from build123d import *

# Parameters (mm, degrees)
SKETCH1_W                    = 235
SKETCH1_H                    = 1200
BASE_FLANGE1_DEPTH           = 1
EDGE_FLANGE2_STRIP_W         = 5.4732
EDGE_FLANGE2_STRIP_H         = 1
EDGE_FLANGE2_STRIP_CUT_DEPTH = 1200
EDGE_FLANGE2_DEPTH           = 1200
EDGE_FLANGE3_DEPTH           = 1200
EDGE_FLANGE4_STRIP_W         = 5.4732
EDGE_FLANGE4_STRIP_H         = 1
EDGE_FLANGE4_STRIP_CUT_DEPTH = 1200
EDGE_FLANGE4_DEPTH           = 1200
EDGE_FLANGE5_DEPTH           = 1200


# Sheet-metal steps are written as plain solids
with BuildPart() as part:
    # Sketch1 → Base-Flange1 (new body)
    with BuildSketch(Plane.XY):
        with Locations((-1020.895638629, 1263.161993769)):
            Rectangle(SKETCH1_W, SKETCH1_H)
    extrude(amount=-BASE_FLANGE1_DEPTH)

    # Edge-Flange2 strip (across the edge) → Edge-Flange2 strip cut (cut)
    with BuildSketch(Plane(origin=(-1138.395638629, 1863.161993769, 0), x_dir=(1, 0, 0), z_dir=(0, -1, 0))):
        with Locations((-1, -0.5)):
            Rectangle(EDGE_FLANGE2_STRIP_W, EDGE_FLANGE2_STRIP_H)
    extrude(amount=EDGE_FLANGE2_STRIP_CUT_DEPTH, mode=Mode.SUBTRACT)

    # Edge-Flange2 section (across the edge) → Edge-Flange2 (add)
    with BuildSketch(Plane(origin=(-1138.395638629, 1863.161993769, 0), x_dir=(1, 0, 0), z_dir=(0, -1, 0))):
        with BuildLine():
            Line((0, 0.7366), (0, 51))
            Line((0, 51), (1, 51))
            Line((1, 51), (1, 0.7366))
            ThreePointArc((1, 0.7366), (1.215745145, 0.215745145), (1.7366, 0))
            Line((1.7366, 0), (1.7366, -1))
            ThreePointArc((1.7366, -1), (0.508638364, -0.491361636), (0, 0.7366))
        make_face()
    extrude(amount=EDGE_FLANGE2_DEPTH)

    # Edge-Flange3 section (across the edge) → Edge-Flange3 (add)
    with BuildSketch(Plane(origin=(-1137.395638629, 1863.161993769, 51.7366), x_dir=(0, 0, -1), z_dir=(0, -1, 0))):
        with BuildLine():
            Line((-1, 0.7366), (-1, 14))
            Line((-1, 14), (0, 14))
            Line((0, 14), (0, 0.7366))
            ThreePointArc((0, 0.7366), (0.215745145, 0.215745145), (0.7366, 0))
            Line((0.7366, 0), (0.7366, -1))
            ThreePointArc((0.7366, -1), (-0.491361636, -0.491361636), (-1, 0.7366))
        make_face()
    extrude(amount=EDGE_FLANGE3_DEPTH)

    # Edge-Flange4 strip (across the edge) → Edge-Flange4 strip cut (cut)
    with BuildSketch(Plane(origin=(-903.395638629, 663.161993769, 0), x_dir=(-1, 0, 0), z_dir=(0, 1, 0))):
        with Locations((-1, -0.5)):
            Rectangle(EDGE_FLANGE4_STRIP_W, EDGE_FLANGE4_STRIP_H)
    extrude(amount=EDGE_FLANGE4_STRIP_CUT_DEPTH, mode=Mode.SUBTRACT)

    # Edge-Flange4 section (across the edge) → Edge-Flange4 (add)
    with BuildSketch(Plane(origin=(-903.395638629, 663.161993769, 0), x_dir=(-1, 0, 0), z_dir=(0, 1, 0))):
        with BuildLine():
            Line((0, 0.7366), (0, 67))
            Line((0, 67), (1, 67))
            Line((1, 67), (1, 0.7366))
            ThreePointArc((1, 0.7366), (1.215745145, 0.215745145), (1.7366, 0))
            Line((1.7366, 0), (1.7366, -1))
            ThreePointArc((1.7366, -1), (0.508638364, -0.491361636), (0, 0.7366))
        make_face()
    extrude(amount=EDGE_FLANGE4_DEPTH)

    # Edge-Flange5 section (across the edge) → Edge-Flange5 (add)
    with BuildSketch(Plane(origin=(-904.395638629, 663.161993769, 67.7366), x_dir=(0, 0, -1), z_dir=(0, 1, 0))):
        with BuildLine():
            Line((-1, 0.7366), (-1, 49))
            Line((-1, 49), (0, 49))
            Line((0, 49), (0, 0.7366))
            ThreePointArc((0, 0.7366), (0.215745145, 0.215745145), (0.7366, 0))
            Line((0.7366, 0), (0.7366, -1))
            ThreePointArc((0.7366, -1), (-0.491361636, -0.491361636), (-1, 0.7366))
        make_face()
    extrude(amount=EDGE_FLANGE5_DEPTH)


solid = part.part
Input: part model. Units: mm. Frame: model coordinates. A direction names the side the tool comes from. Give positions to 0.01 mm unless a question says otherwise; leave off trailing zeros. Write each loop counter-clockwise with the first axis right and the second up, starting at its lowest first coordinate (ties: lowest second). Pieces come first, ordered by that corner, then holes.
Q1. Set-up query: faces 1 (the face through (-930, 1255, 67.737)), 2 (the face through (-903.396, 1255, 33)), 3 (the face through (-1023, 1272, 0)). Return all of +Z, -Z, +X, -X, +Y, -Y with unobstructed straight access to the full face (end or side cutting, diameter ignored); none if empty.
Q2. Section A-A, the plane z = 38.5. Output: boundary loops of the cut face in (x, y), plus the area to 3 significant figures.
Q3. Section D-D, the plane x = -1006. Output: boundary loops of the cut face in (y, z).
Q4. First-contact query: P1, Ø4, axis at x = -1130, y = 1096, coming from the +Z side; P2, Ø10, axis at x = -1057.5, y = 1654.5, coming from the +Z side; P3, Ø1, axis at y = 1635, z = 55.5, coming from the -X side. Flat tips, straight axial feed; report the tip coordinate or a pass-through.
Q5. Pull-direction query (Z, two-part tool) for faces 4 (the face through (-1138.396, 1272, 26)), 5 (the face through (-929, 1255, 68.737)), 6 (the face through (-1137.396, 1272, 26)); classes: pulls with the +Z half, pulls with the -Z half, needs draft (parallel to the pull), parting line crosses it, or undercut.
Q6. Section B-B, the plane x = -943. Output: boundary loops of the cut face in (y, z).
Q7. Section C-C, the plane y = 1551.5. Output: boundary loops of the cut face in (x, z).
Q8. Material intervals for probe 1 along Z at (x, y) = (-932.5, 1653.5); probe 2 along X at (y, z) = (1348.5, 38.5); probe 3 along Z at (x, y) = (-1070, 1383.5), sorted ascending.
Filled in:
1. face 1: -X, +Y, -Y
1. face 2: +Z, -Z, +X, +Y, -Y
1. face 3: +Y, -Y
2. outline: (-1138.4, 663.16) - (-1137.4, 663.16) - (-1137.4, 1863.16) - (-1138.4, 1863.16) - close; (-904.4, 663.16) - (-903.4, 663.16) - (-903.4, 1863.16) - (-904.4, 1863.16) - close
2. area: 2,400 mm2
3. outline: (663.16, -1) - (1863.16, -1) - (1863.16, 0) - (663.16, 0) - close
4. P1: stops at z = 52.74
4. P2: stops at z = 0
4. P3: stops at x = -904.4
5. face 4: needs draft
5. face 5: pulls with the +Z half
5. face 6: undercut
6. outline: (663.16, -1) - (1863.16, -1) - (1863.16, 0) - (663.16, 0) - close; (663.16, 67.74) - (1863.16, 67.74) - (1863.16, 68.74) - (663.16, 68.74) - close
7. outline: (-1138.4, 0.74) arc R1.74 ccw to (-1136.66, -1) - (-905.13, -1) arc R1.74 ccw to (-903.4, 0.74) - (-903.4, 67) arc R1.74 ccw to (-905.13, 68.74) - (-953.4, 68.74) - (-953.4, 67.74) - (-905.13, 67.74) arc R0.74 cw to (-904.4, 67) - (-904.4, 0.74) arc R0.74 cw to (-905.13, 0) - (-1136.66, 0) arc R0.74 cw to (-1137.4, 0.74) - (-1137.4, 51) arc R0.74 cw to (-1136.66, 51.74) - (-1123.4, 51.74) - (-1123.4, 52.74) - (-1136.66, 52.74) arc R1.74 ccw to (-1138.4, 51) - close
8. probe 1: z = -1 to 0, 67.74 to 68.74
8. probe 2: x = -1138.4 to -1137.4, -904.4 to -903.4
8. probe 3: z = -1 to 0
